from build123d import *
from build123d.topology import SkipClean

# Parameters (mm, degrees)
SKETCH_1_R               = 65
EXTRUDE_1_DEPTH          = 72
EXTRUDE_2_DEPTH          = 70
EXTRUDE_2_DEPTH_BACK     = 100
SKETCH_2_R               = 65
SKETCH_3_R               = 45
CUT_EXTRUDE_1_DEPTH      = 228.802546079
CUT_EXTRUDE_3_DEPTH      = 182.642506039
CUT_EXTRUDE_3_DEPTH_BACK = 182.642506039
SKETCH_6_R               = 57.5
CUT_EXTRUDE_4_DEPTH      = 26
SKETCH_7_R               = 62.5
CUT_EXTRUDE_5_DEPTH      = 71
SKETCH_8_R               = 55
CUT_EXTRUDE_6_DEPTH      = 62
PATTERN_CIRCULAR_1_COUNT = 12
PATTERN_CIRCULAR_2_COUNT = 12
SKETCH_18_R              = 1
CUT_EXTRUDE_17_DEPTH     = 32
SKETCH_19_R              = 1
CUT_EXTRUDE_18_DEPTH     = 53
SKETCH_20_R              = 1
CUT_EXTRUDE_19_DEPTH     = 7
CHAMFER_3_SIZE           = 5
SKETCH_29_R              = 50
CUT_EXTRUDE_23_DEPTH     = 8
PATTERN_CIRCULAR_3_COUNT = 10
CUT_EXTRUDE_24_DEPTH     = 20


with BuildPart() as part:
    # 草图1 → 凸台-拉伸1 (new body)
    with BuildSketch(Plane.XY):
        Circle(SKETCH_1_R)
    extrude(amount=EXTRUDE_1_DEPTH)

    # 草图2 → 凸台-拉伸2 (add, two sides: drawn at the far end of the back side and taken through both)
    with BuildSketch(Plane(origin=(0, 0, 0), x_dir=(0, 0, -1), z_dir=(1, 0, 0)).offset(-EXTRUDE_2_DEPTH_BACK)):
        with Locations((-72, 0)):
            Circle(SKETCH_2_R)
    extrude(amount=EXTRUDE_2_DEPTH + EXTRUDE_2_DEPTH_BACK)

    # 草图3 → 切除-拉伸1 (cut, through all)
    with BuildSketch(Plane(origin=(70, 0, 0), x_dir=(0, 0, -1), z_dir=(1, 0, 0))):
        with Locations((-72, 0)):
            Circle(SKETCH_3_R)
    extrude(amount=-CUT_EXTRUDE_1_DEPTH, mode=Mode.SUBTRACT)

    # 草图5 → 切除-拉伸3 (cut, two sides: drawn at the far end of the back side and taken through both)
    with BuildSketch(Plane(origin=(0, 0, 0), x_dir=(1, 0, 0), z_dir=(0, 1, 0)).offset(-CUT_EXTRUDE_3_DEPTH_BACK)):
        Polygon((70, -7), (70, -137), (22.683869545, -137), align=None)
    extrude(amount=CUT_EXTRUDE_3_DEPTH + CUT_EXTRUDE_3_DEPTH_BACK, mode=Mode.SUBTRACT)

    # 草图6 → 切除-拉伸4 (cut)
    with BuildSketch(Plane.ZY.offset(100)):
        with Locations((72, 0)):
            Circle(SKETCH_6_R)
    extrude(amount=-CUT_EXTRUDE_4_DEPTH, mode=Mode.SUBTRACT)

    # 草图7 → 切除-拉伸5 (cut)
    with BuildSketch(Plane(origin=(75, 0, 0), x_dir=(0, 0, -1), z_dir=(1, 0, 0))):
        with Locations((-72, 0)):
            Circle(SKETCH_7_R)
    extrude(amount=-CUT_EXTRUDE_5_DEPTH, mode=Mode.SUBTRACT)

    # 草图8 → 切除-拉伸6 (cut)
    with BuildSketch(Plane(origin=(4, 0, 0), x_dir=(0, 0, -1), z_dir=(1, 0, 0))):
        with Locations((-72, 0)):
            Circle(SKETCH_8_R)
    extrude(amount=-CUT_EXTRUDE_6_DEPTH, mode=Mode.SUBTRACT)

    # 草图9 → M4 螺纹孔1 (revolve, cut)
    with BuildSketch(Plane(origin=(-74, 51, 72), x_dir=(0, 0, 1), z_dir=(0, 1, 0))):
        Polygon((0, 0), (0, 11.091420021), (1.65, 10.1), (1.65, 0), align=None)
    hole_wizard_m4_1 = revolve(axis=Axis((-80.35, 51, 72), (1, 0, 0)), mode=Mode.SUBTRACT)

    # 阵列(圆周)1: M4 螺纹孔1 ×12 about axis
    pattern_circular_1_axis = Axis((0, 0, 72), (1, 0, 0))
    for i in range(1, PATTERN_CIRCULAR_1_COUNT):
        add(hole_wizard_m4_1.rotate(pattern_circular_1_axis, i * 360 / PATTERN_CIRCULAR_1_COUNT), mode=Mode.SUBTRACT)

    # 草图11 → M4 螺纹孔2 (revolve, cut)
    with BuildSketch(Plane(origin=(4, 0, 129), x_dir=(0, 0, -1), z_dir=(0, 1, 0))):
        Polygon((0, 0), (0, 11.091420021), (1.65, 10.1), (1.65, 0), align=None)
    hole_wizard_m4_2 = revolve(axis=Axis((10.35, 0, 129), (-1, 0, 0)), mode=Mode.SUBTRACT)

    # 阵列(圆周)2: M4 螺纹孔2 ×12 about axis
    pattern_circular_2_axis = Axis((0, 0, 72), (1, 0, 0))
    for i in range(1, PATTERN_CIRCULAR_2_COUNT):
        add(hole_wizard_m4_2.rotate(pattern_circular_2_axis, i * 360 / PATTERN_CIRCULAR_2_COUNT), mode=Mode.SUBTRACT)

    # 草图18 → 切除-拉伸17 (cut)
    with BuildSketch(Plane(origin=(75, 0, 0), x_dir=(0, 0, -1), z_dir=(1, 0, 0))):
        with Locations((-72, 63.75)):
            Circle(SKETCH_18_R)
        with Locations((-72, -63.75)):
            Circle(SKETCH_18_R)
    extrude(amount=-CUT_EXTRUDE_17_DEPTH, mode=Mode.SUBTRACT)

    # 草图19 → 切除-拉伸18 (cut)
    with BuildSketch(Plane(origin=(75, 0, 0), x_dir=(0, 0, -1), z_dir=(1, 0, 0))):
        with Locations((-135.75, 0)):
            Circle(SKETCH_19_R)
    extrude(amount=-CUT_EXTRUDE_18_DEPTH, mode=Mode.SUBTRACT)

    # 草图20 → 切除-拉伸19 (cut)
    with BuildSketch(Plane(origin=(75, 0, 0), x_dir=(0, 0, -1), z_dir=(1, 0, 0))):
        with Locations((-8.25, 0)):
            Circle(SKETCH_20_R)
    extrude(amount=-CUT_EXTRUDE_19_DEPTH, mode=Mode.SUBTRACT)

    # 倒角3
    chamfer_3_edges = [part.edges().sort_by_distance(p)[0] for p in [
        (-65, 0, 0),
    ]]
    chamfer(chamfer_3_edges, length=CHAMFER_3_SIZE)

    # 草图27 → M4 螺纹孔4 (revolve, cut)
    with BuildSketch(Plane.YZ.offset(55)):
        Polygon((0, 0), (0, 11.091420021), (1.65, 10.1), (1.65, 0), align=None)
    hole_wizard_m4_4 = revolve(axis=Axis((55, 0, -6.35), (0, 0, 1)), mode=Mode.SUBTRACT)

    # 草图29 → 切除-拉伸23 (cut)
    with BuildSketch(Plane(origin=(0, 0, 0), x_dir=(-1, 0, 0), z_dir=(0, 0, -1))):
        Circle(SKETCH_29_R)
    extrude(amount=-CUT_EXTRUDE_23_DEPTH, mode=Mode.SUBTRACT)

    # 阵列(圆周)3: M4 螺纹孔4 ×10 about axis
    pattern_circular_3_axis = Axis((0, 0, 0), (0, 0, 1))
    for i in range(1, PATTERN_CIRCULAR_3_COUNT):
        add(hole_wizard_m4_4.rotate(pattern_circular_3_axis, i * 360 / PATTERN_CIRCULAR_3_COUNT), mode=Mode.SUBTRACT)

    # 草图30 → 切除-拉伸24 (cut)
    with SkipClean():  # the faces are left unmerged after this step: merging them gives an invalid solid
        with BuildSketch(Plane(origin=(0, 0, 8), x_dir=(-1, 0, 0), z_dir=(0, 0, -1))):
            with BuildLine():
                Line((-22, 44.899888641), (-22, -44.899888641))
                ThreePointArc((-22, -44.899888641), (-50, 0), (-22, 44.899888641))
            make_face()
        extrude(amount=-CUT_EXTRUDE_24_DEPTH, mode=Mode.SUBTRACT)


solid = part.part
CAD build for the part. Positions are in the model's coordinates, mm. A direction names the side the tool comes from. Coordinates: 2 decimals unless noted, no trailing zeros. Write each loop counter-clockwise with the first axis right and the second up, starting at its lowest first coordinate (ties: lowest second). Pieces come first, ordered by that corner, then holes. Notation, with made-up numbers: M 68.5,3 L 102.5,3 A35 ccw 102.5,37 Z; hole C -35,-36.75 d10. An arc over 180 degrees is marked long. Answer as a JSON object with one key per item and string values. Group by question number.
1) Tool access for faces 5 (the face through (15.304, -23.938, 14.266)), 6 (the face through (13, -49, 0)), 7 (the face through (-74, 39, 97)), 8 (the face through (-5, 1, 8)): list every direction of +Z, -Z, +X, -X, +Y, -Y with a clear straight run to the whole face (end or side of a thin tool).
2) Saw through at C-C (z = 104.5). Write the cut outline in (x, y), plus the area to 3 significant figures.
3) Mould opens along X. For faces 1 (the face through (22, 0, 9)), 2 (the face through (-100, -57.5, 67.5)), 3 (the face through (-66, -27, 108)), 4 (the face through (-8.462, 64.447, 23.142)) say: +X half, -X half, draft (parallel to the pull), parting line (faces both ways), or undercut.
4) Saw through at A-A (z = 33). Write the cut outline in (x, y), plus the area to 3 significant figures.
5) Saw through at B-B (y = -6.5). Give the number of separate pieces and of enclosed holes in the cut face, plus the area to 3 significant figures.
6) Wall check: line 1 (Z direction, x = -3.5, y = -28.5); line 2 (Y direction, x = -67, z = 97); line 3 (X direction, y = 46, z = 46). Give the ranges that are in metal, low to high. Write a range as from..to.
7) Pin check, flat tips, straight feed: pin 1 Ø2.5 at (x, y) = (44.5, 32.33) entering from +Z; pin 2 Ø3 at (x, z) = (-80, 17) entering from -Y; pin 3 Ø8 at (x, z) = (-4, 76.5) entering from -Y. Stop position of each tip, or through.
Values follow:
{
 "1": {"face 5": "+X", "face 6": "-Z, +X, -X, +Y, -Y", "face 7": "-X", "face 8": "-Z"},
 "2": {"outline": "M -100,-56.29 L 34.51,-56.29 L 34.51,-53.39 L 4,-53.39 L 4,-44.37 L -58,-44.37 L -58,-31.12 L -74,-31.12 L -74,-47.43 L -100,-47.43 Z; M -100,47.43 L -74,47.43 L -74,31.12 L -58,31.12 L -58,44.37 L 4,44.37 L 4,53.39 L 34.51,53.39 L 34.51,56.29 L -100,56.29 Z", "area": "2,920 mm2"},
 "3": {"face 1": "undercut", "face 2": "-X half", "face 3": "draft", "face 4": "parting line"},
 "4": {"outline": "M -100,-52 L -39,-52 A65 ccw 39,-52 L 60.54,-52 L 60.54,-48.84 L 4,-48.84 L 4,-38.78 L -58,-38.78 L -58,-22.45 L -74,-22.45 L -74,-42.25 L -100,-42.25 Z; M -100,42.25 L -74,42.25 L -74,22.45 L -58,22.45 L -58,38.78 L 4,38.78 L 4,48.84 L 60.54,48.84 L 60.54,52 L 39,52 A65 ccw -39,52 L -100,52 Z", "area": "4,830 mm2"},
 "5": {"separate pieces": "3", "enclosed holes": "0", "area": "2,580 mm2"},
 "6": {"line 1": "z = 8..20.99, 24.29..24.96, 119.04..119.71, 123.01..130.42", "line 2": "y = -60..-45.74, -42.59..-37.42, 37.42..42.59, 45.74..60", "line 3": "x = -74..-58"},
 "7": {"pin 1": "stops at z = 19.29", "pin 2": "stops at y = -36.92", "pin 3": "stops at y = -65"}
}
